Geometry check sheet. Reference: the model listing, model coordinates, mm. A direction names the side the tool comes from. Give positions to 0.01 mm unless a question says otherwise; leave off trailing zeros. Order: outer loops, then holes, each group sorted by start corner. A loop starts at its lowest first (then second) coordinate and runs counter-clockwise, first axis right, second up.
from build123d import *

# Parameters (mm, degrees)
F4_R     = 3.175
F5_DEPTH = 50.8
F7_ANGLE = 113.4
F8_ANGLE = 108.2
F9_ANGLE = 108.8


with BuildPart() as f2:
    # F0 (on Front) → F2 (revolve)
    with BuildSketch(Plane.XZ):
        with BuildLine():
            Line((0, -15.875), (0, 15.875))
            ThreePointArc((0, 15.875), (-15.875, 0), (0, -15.875))
        make_face()
    revolve(axis=Axis((0, 0, 0), (0, 0, 1)))


with BuildPart() as f5:
    # F4 (on offset) → F5 (new body)
    with BuildSketch(Plane.XY.offset(10.16)):
        Circle(F4_R)
    extrude(amount=F5_DEPTH)


with BuildPart() as f7_1:
    # F7: copy of F5
    add(f5.part.rotate(Axis((-36.3165959716, 0, 0), (-1, 0, 0)), F7_ANGLE))


with BuildPart() as f8_1:
    # F8: copy of F7_1
    add(f7_1.part.rotate(Axis((0, 0, -29.0343631059), (0, 0, -1)), F8_ANGLE))


with BuildPart() as f9_1:
    # F9: copy of F8_1
    add(f8_1.part.rotate(Axis((0, 0, -29.0343631059), (0, 0, -1)), F9_ANGLE))


with BuildPart() as f2_1:
    add(f2.part)

    # F10: cut F5, F7_1, F9_1, F8_1
    add(f5.part, mode=Mode.SUBTRACT)
    add(f7_1.part, mode=Mode.SUBTRACT)
    add(f9_1.part, mode=Mode.SUBTRACT)
    add(f8_1.part, mode=Mode.SUBTRACT)


solid = f2_1.part
Item 1: Sectioned sample at B-B (z = -10). Enter the section's corners in (x, y).
Reported:
outline: circle Ø24.66 at (0, 0)
Item 2: Gauge pin test, flat ends, axial feed: pin 1 (8 mm diameter, centred on x = 1.5, y = 12.5, fed in from -Z); pin 2 (1 mm diameter, centred on x = -7.5, y = -4, fed in from -Z); pin 3 (3 mm diameter, centred on y = -10.5, z = -4.5, fed in from -X). Record the tip position at first contact, or that the pin passes through.
Reported:
pin 1: stops at z = -13.35
pin 2: stops at z = -13.71
pin 3: stops at x = -12.39
Item 3: Set-up check for faces 1 (the cylindrical face through (-0.69, -3.1, 12.82)), 2 (the flat face through (-5.565, -7.459, -4.076)): record each of +Z, -Z, +X, -X, +Y, -Y from which the full face is reachable in a straight line by a thin tool's end or side.
Reported:
face 1: +Z
face 2: none
Item 4: Scan lines: L1, parallel to Y at x = 0, z = 12 (3 decimals); L2, parallel to Z at x = 0, y = 8.5; L3, parallel to X at y = 0, z = 11.65 (3 decimals). Record each from-to range of solid material in increasing order.
Reported:
L1: y = -10.393 to -3.175, 3.175 to 10.393
L2: z = -13.41 to -7.14, -5.94 to 13.41
L3: x = -10.784 to -3.175, 3.175 to 10.784
Item 5: Sectioned sample at A-A (x = -1). Enter the section's corners in (y, z), and give its area (3 significant figures).
Reported:
outline: (-3.01, 10.16) - (-3.01, 15.55) arc R15.84 ccw (long way) to (13.08, -8.94) - (8.13, -6.8) - (10.52, -1.27) - (15.47, -3.41) arc R15.84 ccw to (3.01, 15.55) - (3.01, 10.16) - close
area: 721 mm2
Item 6: Sectioned sample at C-C (y = 4.5). Enter the section's corners in (x, z).
Reported:
outline: circle Ø30.45 at (0, 0)
